The listing builds one solid part. Answer for the finished solid, in the listing's coordinates (mm). Face numbers are marked on the shaded views. Give positions to 0.01 mm unless a question says otherwise; leave off trailing zeros. Loops run counter-clockwise (first coordinate to the right, second up) from the corner with the lowest first, then second, coordinate; pieces in that order, holes last. Notation, with made-up numbers: M -5.5,47 L 33.5,47 A21 cw 33.5,82 Z; hole C -32.5,10.5 d11. An arc over 180 degrees is marked long. Use one line per item in the form item = value. Start each with the question number.
1. Each of these flat-tipped pins is pushed along its axis until it touches: pin 1 Ø1.6 at (x, y) = (8.5, 3.5) entering from +Z; pin 2 Ø8 at (x, z) = (-10, -10.5) entering from +Y; pin 3 Ø1 at (x, y) = (-6, 4) entering from +Z. Where does it stop, or does it pass through?
2. The mould has two halves that part along X. Classify the marked faces 1, 2, 3 and 4: released by +X, released by -X, zero draft, split by the parting line, or undercut.
3. Straight lines are drawn through the part: line 1 (X direction, y = 1.25, z = -4); line 2 (X direction, y = 2.75, z = 16.5); line 3 (Z direction, x = 12.5, y = 4.75). For each, find the intervals that lie inside material, in ascending order. Write a range as from..to.
4. The part is cut by section A-A (y = 3). Write down the section's boundary in (x, z), and give its area (3 significant figures).
5. The part is cut by section C-C (z = 6.5). Write down the section's boundary in (x, y).
6. The part is cut by section B-B (x = 9). Write down the section's boundary in (y, z), and give its area (3 significant figures).
7. The part is cut by section D-D (x = 2). Write down the section's boundary in (y, z).
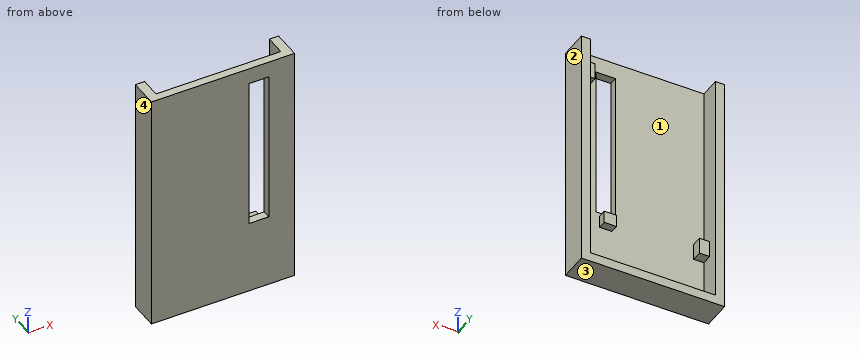
Autodesk Inventor part; units mm, degrees
ref_plane "YZ Plane" through (0, 0, 0) normal (1, 0, 0) x (0, 1, 0)
ref_plane "XZ Plane" through (0, 0, 0) normal (0, 1, 0) x (-1, 0, 0)
ref_plane "XY Plane" through (0, 0, 0) normal (0, 0, 1) x (1, 0, 0)
sketch "Sketch1" plane through (0, 0, 0) normal (0, 1, 0) x (-1, 0, 0)
  line L0 (-17.5, -29.75) -> (17.5, -29.75)
  line L1 (17.5, -29.75) -> (17.5, 29.75)
  line L2 (17.5, 29.75) -> (-17.5, 29.75)
  line L3 (-17.5, 29.75) -> (-17.5, -29.75)
  line L4 (-17.5, -29.75) -> (17.5, 29.75) construction
  line L5 (17.5, -29.75) -> (-17.5, 29.75) construction
  point P0 (0, 0)
  dimension "d0" = 59.5
  dimension "d1" = 35
extrude "Extrusion1" add sketch "Sketch1" along normal blind 7
sketch "Sketch2" plane through (0, 7, 0) normal (0, 1, 0) x (1, 0, 0)
  line L0 (-17.5, -29.75) -> (17.5, -29.75)
  line L1 (15.25, -29.75) -> (-15.25, -29.75)
  line L2 (-15.25, -29.75) -> (-15.25, 27.5)
  line L3 (-15.25, 27.5) -> (15.25, 27.5)
  line L4 (15.25, 27.5) -> (15.25, -29.75)
  line L5 (17.5, -29.75) -> (17.5, 29.75)
  line L6 (17.5, 29.75) -> (-17.5, 29.75)
  line L7 (-17.5, 29.75) -> (-17.5, -29.75)
  point P0 (0, 0)
  point P1 (-15.25, -29.75)
  dimension "d4" = 2.25
  dimension "d5" = 2.25
  dimension "d6" = 2.25
extrude "Extrusion2" cut sketch "Sketch2" against normal blind 5 contours L2 L3 L4 L0
sketch "Sketch3" plane through (0, 2, 0) normal (0, 1, 0) x (1, 0, 0)
  line L0 (10.25, 15.5) -> (7.25, 15.5)
  line L1 (7.25, 15.5) -> (7.25, 12.5)
  line L2 (7.25, 12.5) -> (10.25, 12.5)
  line L3 (10.25, 12.5) -> (10.25, 15.5)
  line L4 (-15.25, 27.5) -> (15.25, 27.5)
  line L5 (15.25, 27.5) -> (15.25, -29.75)
  line L6 (15.25, -25.75) -> (12.75, -25.75)
  line L7 (12.75, -25.75) -> (12.75, -21.75)
  line L8 (12.75, -21.75) -> (15.25, -21.75)
  line L9 (15.25, -21.75) -> (15.25, -25.75)
  line L10 (-15.25, -29.75) -> (-15.25, 27.5)
  line L11 (-15.25, 11.5) -> (-12.75, 11.5)
  line L12 (-12.75, 11.5) -> (-12.75, 15.5)
  line L13 (-12.75, 15.5) -> (-15.25, 15.5)
  line L14 (-15.25, 15.5) -> (-15.25, 11.5)
  line L15 (15.25, -29.75) -> (-15.25, -29.75)
  point P0 (0, 0)
  point P1 (15.25, -21.75)
  dimension "d9" = 3
  dimension "d10" = 3
  dimension "d21" = 12
  dimension "d22" = 5
  dimension "d23" = 2.5
  dimension "d24" = 4
  dimension "d25" = 4
  dimension "d26" = 2.5
  dimension "d27" = 12
  dimension "d28" = 4
extrude "Extrusion3" add sketch "Sketch3" along normal blind 2 contours L3 L2 L1 L0
extrude "Extrusion4" add sketch "Sketch3" along normal blind 2.5 contours L13 L12 L11 L10 | L5 L6 L7 L8
sketch "Sketch4" plane through (0, 2, 0) normal (0, 1, 0) x (1, 0, 0)
  line L0 (11.1804, 11.7081) -> (6.3882, 11.7081)
  line L1 (6.3882, 11.7081) -> (6.3882, -25.8012)
  line L2 (6.3882, -25.8012) -> (11.1804, -25.8012)
  line L3 (11.1804, -25.8012) -> (11.1804, 11.7081)
  point P0 (0, 0)
extrude "Extrusion5" cut sketch "Sketch4" against normal through all
equation "\"d5\" = d4"
equation "\"d6\" = d4"
equation "\"d25\" = d24"
equation "\"d26\" = d23"
properties part number "CROC Gluing Form V2"
Derived:
q1.pin_1 = -12.5
q1.pin_2 = 4.5
q1.pin_3 = -27.5
q2.face_1 = undercut
q2.face_2 = released by +X
q2.face_3 = zero draft
q2.face_4 = released by -X
q3.line_1 = -17.5..6.39, 11.18..17.5
q3.line_2 = -17.5..-15.25, 15.25..17.5
q3.line_3 = -29.75..-27.5
q4.outline = M -17.5,-29.75 L 17.5,-29.75 L 17.5,29.75 L 15.25,29.75 L 15.25,25.75 L 12.75,25.75 L 12.75,21.75 L 15.25,21.75 L 15.25,-27.5 L -15.25,-27.5 L -15.25,-15.5 L -12.75,-15.5 L -12.75,-11.5 L -15.25,-11.5 L -15.25,29.75 L -17.5,29.75 Z; M 7.25,-15.5 L 10.25,-15.5 L 10.25,-12.5 L 7.25,-12.5 Z
q4.area = 365 mm2
q5.outline = M -17.5,0 L 6.39,0 L 6.39,2 L -15.25,2 L -15.25,7 L -17.5,7 Z; M 11.18,0 L 17.5,0 L 17.5,7 L 15.25,7 L 15.25,2 L 11.18,2 Z
q6.outline = M 0,-29.75 L 7,-29.75 L 7,-27.5 L 2,-27.5 L 2,-15.5 L 4,-15.5 L 4,-12.5 L 2,-12.5 L 2,-11.71 L 0,-11.71 Z; M 0,25.8 L 2,25.8 L 2,29.75 L 0,29.75 Z
q6.area = 61.2 mm2
q7.outline = M 0,-29.75 L 7,-29.75 L 7,-27.5 L 2,-27.5 L 2,29.75 L 0,29.75 Z
